The drawing under review shows one solid part. Ordinate dimensions are in mm from its lowest x, y, z. Coordinates: 2 decimals unless noted, no trailing zeros. Write each loop counter-clockwise with the first axis right and the second up, starting at its lowest first coordinate (ties: lowest second). Pieces come first, ordered by that corner, then holes.
Q1. Add section D-D, the plane x = 6.75. Give the boundary of the cut face in (y, z) (1 decimal).
Q2. Clearance check with flat-ended pins moving along their axes: pin 1 Ø1.5 at (x, y) = (7.5, 21) entering from -Z; pin 2 Ø3.5 at (y, z) = (21.96, 6) entering from -X; pin 3 Ø3 at (x, z) = (3.5, 2.5) entering from +Y (1 decimal); pin 4 Ø3 at (x, z) = (4, 5) entering from -Y. State where each tip first meets the part, or that it passes through.
Q3. Add section A-A, the plane x = 4.5. Give the boundary of the cut face in (y, z), plus the area to 3 significant figures.
Q4. To check wall thickness, follow probe 1 along X at (y, z) = (7.5, 6); probe 2 along Y at (x, z) = (6.75, 6); probe 3 along X at (y, z) = (5.75, 7.75) (1 decimal). State the ranges of each line that lie inside material, in increasing order.
Q5. The part is to be moulded in two halves that separate along X. For the marked faces 1, 2, 3 and 4, say which applies: +X half, -X half, draft (parallel to the pull), parting line (faces both ways), or undercut.
Q6. Add section B-B, the plane z = 6. Give the boundary of the cut face in (x, y), plus the area to 3 significant figures.
Q7. Add section C-C, the plane y = 3.5. Give the boundary of the cut face in (x, z).
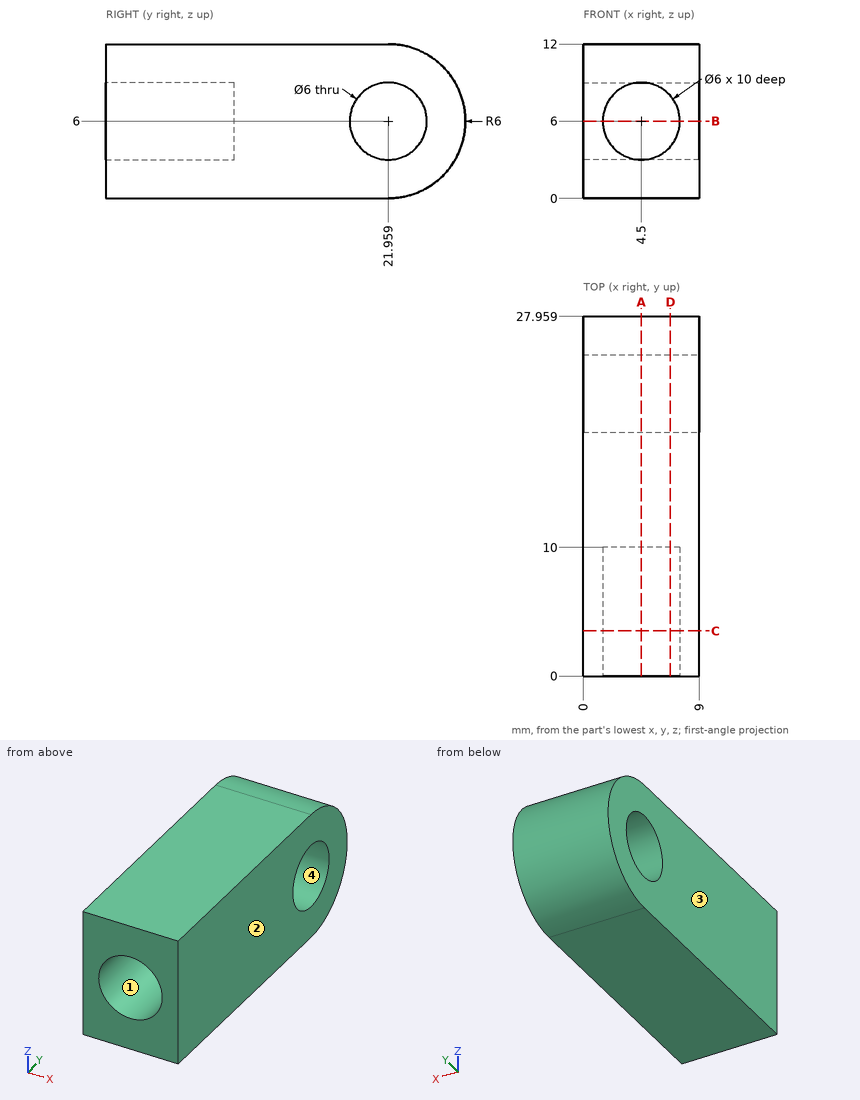
Here are the results:
1. outline: (0, 0) - (22, 0) arc R6 ccw to (22, 12) - (0, 12) - (0, 8) - (10, 8) - (10, 4) - (0, 4) - close; hole circle Ø6 at (22, 6)
2. pin 1: stops at z = 0
2. pin 2: passes through
2. pin 3: stops at y = 27.6
2. pin 4: stops at y = 10
3. outline: (0, 0) - (21.96, 0) arc R6 ccw to (21.96, 12) - (0, 12) - (0, 9) - (10, 9) - (10, 3) - (0, 3) - close; hole circle Ø6 at (21.96, 6)
3. area: 232 mm2
4. probe 1: x = 0 to 1.5, 7.5 to 9
4. probe 2: y = 10 to 18.96, 24.96 to 27.96
4. probe 3: x = 0 to 2.1, 6.9 to 9
5. face 1: undercut
5. face 2: +X half
5. face 3: -X half
5. face 4: draft
6. outline: (0, 0) - (1.5, 0) - (1.5, 10) - (7.5, 10) - (7.5, 0) - (9, 0) - (9, 18.96) - (0, 18.96) - close; (0, 24.96) - (9, 24.96) - (9, 27.96) - (0, 27.96) - close
6. area: 138 mm2
7. outline: (0, 0) - (9, 0) - (9, 12) - (0, 12) - close; hole circle Ø6 at (4.5, 6)
